from build123d import *

# Parameters (mm, degrees)
SKETCH1_R           = 2
BOSS_EXTRUDE1_DEPTH = 52
SKETCH2_R           = 5
BOSS_EXTRUDE2_DEPTH = 1
SKETCH3_W           = 7
SKETCH3_H           = 1
BOSS_EXTRUDE3_DEPTH = 3
FILLET1_R           = 1


with BuildPart() as part:
    # Sketch1 → Boss-Extrude1 (new body)
    with BuildSketch(Plane(origin=(0, 0, 0), x_dir=(1, 0, 0), z_dir=(0, 1, 0))):
        with Locations(Location((0, 0, 0), (0, 0, 90))):
            Circle(SKETCH1_R)
    extrude(amount=BOSS_EXTRUDE1_DEPTH)

    # Sketch2 → Boss-Extrude2 (add)
    with BuildSketch(Plane.XZ):
        with Locations(Location((0, 0, 0), (0, 0, 270))):
            Circle(SKETCH2_R)
    extrude(amount=-BOSS_EXTRUDE2_DEPTH)

    # Sketch3 → Boss-Extrude3 (add)
    with BuildSketch(Plane(origin=(0, 52, 0), x_dir=(1, 0, 0), z_dir=(0, 1, 0))):
        Rectangle(SKETCH3_W, SKETCH3_H)
    extrude(amount=BOSS_EXTRUDE3_DEPTH)

    # Fillet1
    # the kernel refuses this fillet: 1 mm, written as the material it takes off along each edge
    with BuildSketch(Plane(origin=(3.5, 55, 3), x_dir=(0, -1, 0), z_dir=(0, 0, -1)), Plane(origin=(-3.5, 55, -3), x_dir=(0, -1, 0), z_dir=(0, 0, 1))) as fillet1_piece_1:
        with BuildLine():
            CenterArc((FILLET1_R, FILLET1_R), FILLET1_R, 180, 90)
            Line((0, FILLET1_R), (0, 0))
            Line((0, 0), (FILLET1_R, 0))
        make_face()
    extrude(amount=6, mode=Mode.SUBTRACT)
    with BuildSketch(Plane(origin=(6, 55, -0.5), x_dir=(0, -1, 0), z_dir=(-1, 0, 0)), Plane(origin=(-6, 55, 0.5), x_dir=(0, -1, 0), z_dir=(1, 0, 0))) as fillet1_piece_2:
        with BuildLine():
            CenterArc((FILLET1_R, FILLET1_R), FILLET1_R, 180, 90)
            Line((0, FILLET1_R), (0, 0))
            Line((0, 0), (FILLET1_R, 0))
        make_face()
    extrude(amount=12, mode=Mode.SUBTRACT)


solid = part.part
The model under review builds one solid part; all positions refer to its coordinate system, in mm. A direction names the side the tool comes from. Round coordinates to 2 decimals unless told otherwise and drop trailing zeros. Loops run counter-clockwise (first coordinate to the right, second up) from the corner with the lowest first, then second, coordinate; pieces in that order, holes last. Notation, with made-up numbers: M -0.75,-36.75 L 38.25,-36.75 A29 ccw 38.25,-2.75 Z; hole C 28.25,-10.5 d1. An arc over 180 degrees is marked long. Answer as a JSON object with one key per item and string values.
Item 1: We need section C-C, the plane z = 1.5. State the section outline as (x, y) points, and give its area (3 significant figures).
Check sheet entries:
{"outline": "M -4.77,0 L 4.77,0 L 4.77,1 L 1.32,1 L 1.32,52 L -1.32,52 L -1.32,1 L -4.77,1 Z", "area": "144 mm2"}
Item 2: Clearance check with flat-ended pins moving along their axes: P1, Ø6, axis at y = 47.5, z = 3, coming from the -X side; P2, Ø4, axis at x = 0.5, y = 24, coming from the +Z side; P3, Ø1.7, axis at x = 0, z = 1.5, coming from the +Y side. State where each tip first meets the part, or that it passes through.
Check sheet entries:
{"P1": "x = -2", "P2": "z = 2", "P3": "y = 52"}
Item 3: Tool access review of faces 5 (the face through (3.5, 53, 0)), 6 (the face through (0, 53, 0.5)), 7 (the face through (0, 53, -0.5)), 8 (the face through (-3.5, 53, 0)): name each direction out of +Z, -Z, +X, -X, +Y, -Y from which nothing blocks a thin tool from reaching the whole face with its end or side.
Check sheet entries:
{"face 5": "+Z, -Z, +X, +Y", "face 6": "+Z, +X, -X, +Y", "face 7": "-Z, +X, -X, +Y", "face 8": "+Z, -Z, -X, +Y"}
Item 4: For line 1 along Y through (x, z) = (-2.25, 2.25); line 2 along Z through (x, y) = (-0.5, 33), list the stretches that pass through material, from the lowest coordinate up.
Check sheet entries:
{"line 1": "0 to 1", "line 2": "-1.94 to 1.94"}
Item 5: The part is to be moulded in two halves that separate along Y. For faces 1 (the face through (-3, 52, 0)), 2 (the face through (-4.88, 0.49, 1.08)), 3 (the face through (3, 52, 0)), 4 (the face through (0, 52, 1)), say which applies: +Y half, -Y half, draft (parallel to the pull), parting line (faces both ways), or undercut.
Check sheet entries:
{"face 1": "undercut", "face 2": "draft", "face 3": "undercut", "face 4": "+Y half"}
Item 6: We need section B-B, the plane x = 2.5. State the section outline as (y, z) points, and give its area (3 significant figures).
Check sheet entries:
{"outline": "M 0,-4.33 L 1,-4.33 L 1,4.33 L 0,4.33 Z; M 52,-0.5 L 54,-0.5 A1 ccw 54.87,0 A1 ccw 54,0.5 L 52,0.5 Z", "area": "11.3 mm2"}
Item 7: We need section A-A, the plane x = 0. State the section outline as (y, z) points, and give its area (3 significant figures).
Check sheet entries:
{"outline": "M 0,-5 L 1,-5 L 1,-2 L 52,-2 L 52,-0.5 L 54,-0.5 A1 ccw 54.87,0 A1 ccw 54,0.5 L 52,0.5 L 52,2 L 1,2 L 1,5 L 0,5 Z", "area": "217 mm2"}
Item 8: We need section D-D, the plane y = 20. State the section outline as (x, z) points, and give its area (3 significant figures).
Check sheet entries:
{"outline": "C 0,0 d4", "area": "12.6 mm2"}
